from build123d import *

# Parameters (mm, degrees)
BOSS_EXTRUDE1_DEPTH = 4


with BuildPart() as part:
    # Sketch1 → Boss-Extrude1 (new body)
    with BuildSketch(Plane(origin=(0, 0, 0), x_dir=(-1, 0, 0), z_dir=(0, 1, 0))):
        Polygon((0, 0), (0, 150), (-190, 150), (-190, -150), (-40, -150), align=None)
        with BuildLine():
            Line((-97.1, 142.9), (-97.1, 117.1))
            ThreePointArc((-97.1, 117.1), (-95, 115), (-92.9, 117.1))
            Line((-92.9, 117.1), (-92.9, 142.9))
            ThreePointArc((-92.9, 142.9), (-95, 145), (-97.1, 142.9))
        make_face(mode=Mode.SUBTRACT)
        with BuildLine():
            Line((-42.9, 142.9), (-42.9, 117.1))
            ThreePointArc((-42.9, 117.1), (-45, 115), (-47.1, 117.1))
            Line((-47.1, 117.1), (-47.1, 142.9))
            ThreePointArc((-47.1, 142.9), (-45, 145), (-42.9, 142.9))
        make_face(mode=Mode.SUBTRACT)
    extrude(amount=BOSS_EXTRUDE1_DEPTH)


solid = part.part
Here's how the part is built. I have some questions about the finished solid (model axes, mm). Coordinates: 2 decimals unless noted, no trailing zeros. Loops run counter-clockwise (first coordinate to the right, second up) from the corner with the lowest first, then second, coordinate; pieces in that order, holes last.
1. For P1, Ø6, axis at x = 78, z = -44.5, coming from the -Y side, with a flat end and sliding along its axis, tell me the tip position at first contact or that it passes through.
2. I need wall thicknesses on L1, parallel to X at y = 3.3, z = 118; L2, parallel to X at y = 3.7, z = -115.5; L3, parallel to X at y = 0.2, z = -68.5. Which ranges of each line are inside material? Lowest first, please.
3. Imagine slicing it at C-C, the plane z = -51. Please give me the cut outline in (x, y).
4. Imagine slicing it at A-A, the plane y = 1.95. Please give me the cut outline in (x, z), and give its area (3 significant figures).
5. Imagine slicing it at B-B, the plane z = -120. Please give me the cut outline in (x, y), and give its area (3 significant figures).
Taken from the geometry:
1. P1: stops at y = 0
2. L1: x = 0 to 42.9, 47.1 to 92.9, 97.1 to 190
2. L2: x = 30.8 to 190
2. L3: x = 18.27 to 190
3. outline: (13.6, 0) - (190, 0) - (190, 4) - (13.6, 4) - close
4. outline: (0, 0) - (40, -150) - (190, -150) - (190, 150) - (0, 150) - close; hole (42.9, 117.1) arc R2.1 ccw to (47.1, 117.1) - (47.1, 142.9) arc R2.1 ccw to (42.9, 142.9) - close; hole (92.9, 117.1) arc R2.1 ccw to (97.1, 117.1) - (97.1, 142.9) arc R2.1 ccw to (92.9, 142.9) - close
4. area: 53,800 mm2
5. outline: (32, 0) - (190, 0) - (190, 4) - (32, 4) - close
5. area: 632 mm2
